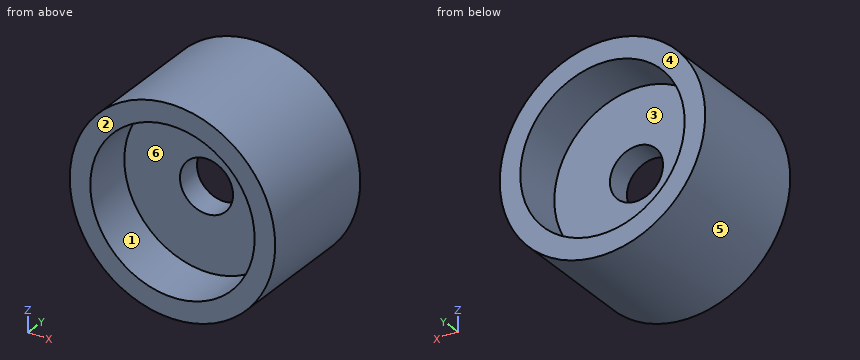
Autodesk Inventor part; units mm, degrees
ref_plane "YZ Plane" through (0, 0, 0) normal (1, 0, 0) x (0, 1, 0)
ref_plane "XZ Plane" through (0, 0, 0) normal (0, 1, 0) x (-1, 0, 0)
ref_plane "XY Plane" through (0, 0, 0) normal (0, 0, 1) x (1, 0, 0)
sketch "Sketch1" plane through (0, 0, 0) normal (0, 1, 0) x (-1, 0, 0)
  circle A0 centre (0, 0) radius 12
  dimension "d1" = 24
extrude "Extrusion1" add sketch "Sketch1" along normal blind 15
sketch "Sketch2" plane through (0, 15, 0) normal (0, 1, 0) x (1, 0, 0)
  circle A0 centre (0, 0) radius 9.6
  dimension "d4" = 19.2
extrude "Extrusion2" cut sketch "Sketch2" against normal blind 6
sketch "Sketch3" plane through (0, 0, 0) normal (0, -1, 0) x (1, 0, 0)
  circle A0 centre (0, 0) radius 9.6
  dimension "d7" = 19.2
extrude "Extrusion3" cut sketch "Sketch3" against normal blind 6
sketch "Sketch4" plane through (0, 9, 0) normal (0, 1, 0) x (1, 0, 0)
  circle A0 centre (0, 0) radius 3.1
  dimension "d10" = 6.2
extrude "Extrusion4" cut sketch "Sketch4" against normal blind 6
properties part number "Belt tensor"
Verification items for the finished model (mm, model axes). Face numbers are marked on the shaded views. A direction names the side the tool comes from. Give positions to 0.01 mm unless a question says otherwise; leave off trailing zeros. Loops run counter-clockwise (first coordinate to the right, second up) from the corner with the lowest first, then second, coordinate; pieces in that order, holes last.
1) Thickness scan on line 1 along Z through (x, y) = (0, 10.85); line 2 along Y through (x, z) = (-7, 4.5); line 3 along Z through (x, y) = (-5.5, 4). Record the ranges inside material, lowest first.
2) Draft check along X on the marked faces 4, 5 and 6. Enter one of: pulls with the +X half, pulls with the -X half, needs draft (parallel to the pull), parting line crosses it, or undercut.
3) Depth check by flat-ended pin: pin 1 Ø5 at (x, y) = (5, 2) entering from -Z; pin 2 Ø8 at (x, y) = (8, 12.5) entering from -Z; pin 3 Ø5 at (y, z) = (1.5, 3.5) entering from -X. Enter the tip coordinate at first touch or a pass-through.
4) Sectioned sample at B-B, the plane x = 0. Enter the section's corners in (y, z).
5) Sectioned sample at C-C, the plane y = 13.5. Enter the section's corners in (x, z), then the cut area to 3 significant figures.
6) Set-up check for the marked faces 1, 2 and 3: record each of +Z, -Z, +X, -X, +Y, -Y from which the full face is reachable in a straight line by a thin tool's end or side.
7) Sectioned sample at D-D, the plane x = 8. Enter the section's corners in (y, z).
8) Sectioned sample at A-A, the plane z = 0. Enter the section's corners in (x, y).
Answers:
1. line 1: z = -12 to -9.6, 9.6 to 12
1. line 2: y = 6 to 9
1. line 3: z = -10.67 to -7.87, 7.87 to 10.67
2. face 4: needs draft
2. face 5: parting line crosses it
2. face 6: undercut
3. pin 1: stops at z = -11.74
3. pin 2: stops at z = -11.31
3. pin 3: stops at x = -11.96
4. outline: (0, -12) - (15, -12) - (15, -9.6) - (9, -9.6) - (9, -3.1) - (6, -3.1) - (6, -9.6) - (0, -9.6) - close; (0, 9.6) - (6, 9.6) - (6, 3.1) - (9, 3.1) - (9, 9.6) - (15, 9.6) - (15, 12) - (0, 12) - close
5. outline: circle Ø24 at (0, 0); hole circle Ø19.2 at (0, 0)
5. area: 163 mm2
6. face 1: -Y
6. face 2: +Z, -Z, +X, -X, -Y
6. face 3: +Y
7. outline: (0, -8.94) - (15, -8.94) - (15, -5.31) - (9, -5.31) - (9, 5.31) - (15, 5.31) - (15, 8.94) - (0, 8.94) - (0, 5.31) - (6, 5.31) - (6, -5.31) - (0, -5.31) - close
8. outline: (-12, 0) - (-9.6, 0) - (-9.6, 6) - (-3.1, 6) - (-3.1, 9) - (-9.6, 9) - (-9.6, 15) - (-12, 15) - close; (3.1, 6) - (9.6, 6) - (9.6, 0) - (12, 0) - (12, 15) - (9.6, 15) - (9.6, 9) - (3.1, 9) - close
